```python
from build123d import *

# Parameters (mm, degrees)
SCHIZZO1_W                   = 100
SCHIZZO1_H                   = 100
ESTRUSIONE_ESTRUSIONE1_DEPTH = 5
SCHIZZO2_R                   = 10
SCHIZZO2_W                   = 20
SCHIZZO2_H                   = 20
ESTRUSIONE_ESTRUSIONE2_DEPTH = 10
ESTRUSIONE_ESTRUSIONE3_DEPTH = 20
NERVATURA6_REACH             = 116.564
SCHIZZO17_WALL_W             = 254.559533776
SCHIZZO17_WALL_H             = 5
NERVATURA7_REACH             = 116.564
SCHIZZO19_WALL_W             = 244.96518431
SCHIZZO19_WALL_H             = 5


with BuildPart() as part:
    # Schizzo1 → Estrusione-Estrusione1 (new, symmetric)
    with BuildSketch(Plane.XY):
        with Locations((50, 50)):
            Rectangle(SCHIZZO1_W, SCHIZZO1_H)
    extrude(amount=ESTRUSIONE_ESTRUSIONE1_DEPTH, both=True)

    # Schizzo2 → Estrusione-Estrusione2 (add)
    with BuildSketch(Plane.XY.offset(5)):
        with Locations(Location((50, 85, 0), (0, 0, 180))):
            Circle(SCHIZZO2_R)
        with Locations((50, 17.098606554)):
            Rectangle(SCHIZZO2_W, SCHIZZO2_H)
        with Locations((85, 50)):
            Rectangle(SCHIZZO2_W, SCHIZZO2_H)
        with Locations(Location((15, 50, 0), (0, 0, 180))):
            Circle(SCHIZZO2_R)
    extrude(amount=ESTRUSIONE_ESTRUSIONE2_DEPTH)

    # Schizzo2_3 → Estrusione-Estrusione3 (add)
    with BuildSketch(Plane.XY.offset(5)):
        with BuildLine():
            Line((57, 42.858571571), (57, 57.141428429))
            ThreePointArc((57, 57.141428429), (40, 50), (57, 42.858571571))
        make_face()
    extrude(amount=ESTRUSIONE_ESTRUSIONE3_DEPTH)

    # Schizzo17 wall → Nervatura6 (add, up to next)
    with BuildSketch(Plane(origin=(66, 50, 17.5), x_dir=(-0.768221279597, 0, 0.640184399664), z_dir=(-0.640184399664, 0, -0.768221279597)), mode=Mode.PRIVATE) as nervatura6_sk1:
        Rectangle(SCHIZZO17_WALL_W, SCHIZZO17_WALL_H)
    nervatura6_tool1 = extrude(nervatura6_sk1.sketch, amount=NERVATURA6_REACH, mode=Mode.PRIVATE) - part.part
    add(nervatura6_tool1.solids().sort_by_distance((66, 50, 17.5))[0])

    # Schizzo19 wall → Nervatura7 (add, up to next)
    with BuildSketch(Plane(origin=(50, 33.549303277, 17.5), x_dir=(0, 0.932424174937, 0.361365684583), z_dir=(0, 0.361365684583, -0.932424174937)), mode=Mode.PRIVATE) as nervatura7_sk1:
        Rectangle(SCHIZZO19_WALL_W, SCHIZZO19_WALL_H)
    nervatura7_tool1 = extrude(nervatura7_sk1.sketch, amount=NERVATURA7_REACH, mode=Mode.PRIVATE) - part.part
    add(nervatura7_tool1.solids().sort_by_distance((50, 33.549303277, 17.5))[0])


solid = part.part
```
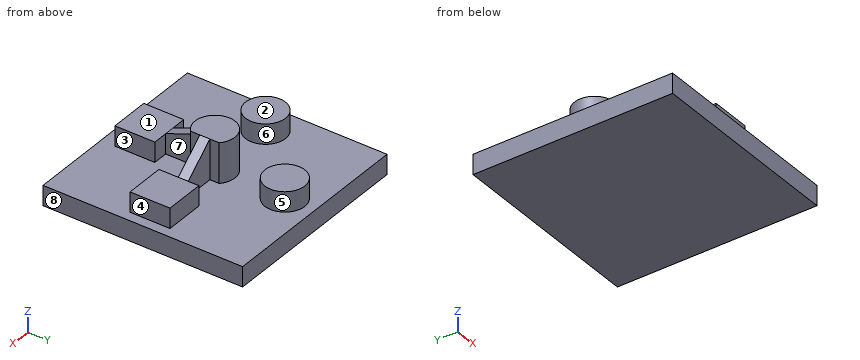
CAD build for the part. Positions are in the model's coordinates, mm. Face numbers are marked on the shaded views. A direction names the side the tool comes from. Round coordinates to 2 decimals unless told otherwise and drop trailing zeros. Write each loop counter-clockwise with the first axis right and the second up, starting at its lowest first coordinate (ties: lowest second). Pieces come first, ordered by that corner, then holes. Notation, with made-up numbers: (-39.5, -30.5) - (-11.5, -30.5) arc R13 ccw to (-11.5, -15.5) - close; hole circle Ø7 at (-11.5, 23). An arc over 180 degrees is marked (long way). Return JSON: item names as keys, results as strings. Group by question number.
Item 1: Band-saw the part on A-A on z = 6.5. List the corners of the cut face in (x, y), plus the area to 3 significant figures.
Item 2: Flat gauge pins, fed straight in: pin 1 Ø6 at (x, y) = (54, 17) entering from +Z; pin 2 Ø4 at (x, z) = (26, 9) entering from -Y; pin 3 Ø8 at (x, z) = (55, 9.5) entering from -Y. Where does each tip first touch, or does it go through?
Item 3: Mould opens along Y. For the marked faces 6, 7 and 8 say: +Y half, -Y half, draft (parallel to the pull), parting line (faces both ways), or undercut.
Item 4: Probe probe 1 along X at (y, z) = (56.5, 14); probe 2 along Z at (x, y) = (37, 35.5); probe 3 along X at (y, z) = (34, 7). List the from-to ranges inside material, lowest first.
Item 5: Band-saw the part on B-B on y = 50. List the corners of the cut face in (x, z).
Item 6: 3-axis set-ups, long thin cutter, end or side, ignore diameter. For the marked faces 1, 2, 3, 4 and 5: which of +Z, -Z, +X, -X, +Y, -Y reach the whole face in a straight line?
Item 7: Band-saw the part on C-C on x = 50. List the corners of the cut face in (y, z), plus the area to 3 significant figures.
Item 8: Band-saw the part on D-D on x = 15. List the corners of the cut face in (y, z).
Resolved:
{
 "1": {"outline": "circle Ø20 at (15, 50); (40, 7.1) - (60, 7.1) - (60, 27.1) - (52.5, 27.1) - (52.5, 40.32) arc R10 ccw to (57, 42.86) - (57, 47.5) - (75, 47.5) - (75, 40) - (95, 40) - (95, 60) - (75, 60) - (75, 52.5) - (57, 52.5) - (57, 57.14) arc R10 ccw (long way) to (47.5, 40.32) - (47.5, 27.1) - (40, 27.1) - close; circle Ø20 at (50, 85)", "area": "1,870 mm²"},
 "2": {"pin 1": "stops at z = 15", "pin 2": "stops at y = 45.64", "pin 3": "stops at y = 7.1"},
 "3": {"face 6": "parting line", "face 7": "undercut", "face 8": "draft"},
 "4": {"probe 1": "x = 7.4 to 22.6, 42.4 to 57, 75 to 95", "probe 2": "z = -5 to 5", "probe 3": "x = 47.5 to 52.5"},
 "5": {"outline": "(0, -5) - (100, -5) - (100, 5) - (95, 5) - (95, 15) - (75, 15) - (75, 10) - (57, 25) - (40, 25) - (40, 5) - (25, 5) - (25, 15) - (5, 15) - (5, 5) - (0, 5) - close"},
 "6": {"face 1": "+Z, +X, -X, -Y", "face 2": "+Z, -X, +Y, -Y", "face 3": "+Z, +X, -Y", "face 4": "+Z, +X, +Y, -Y", "face 5": "+Z"},
 "7": {"outline": "(0, -5) - (100, -5) - (100, 5) - (95, 5) - (95, 15) - (75, 15) - (75, 5) - (60, 5) - (60, 25) - (40, 25) - (40, 20) - (27.1, 15) - (7.1, 15) - (7.1, 5) - (0, 5) - close", "area": "1,960 mm²"},
 "8": {"outline": "(0, -5) - (100, -5) - (100, 5) - (60, 5) - (60, 15) - (40, 15) - (40, 5) - (0, 5) - close"}
}
